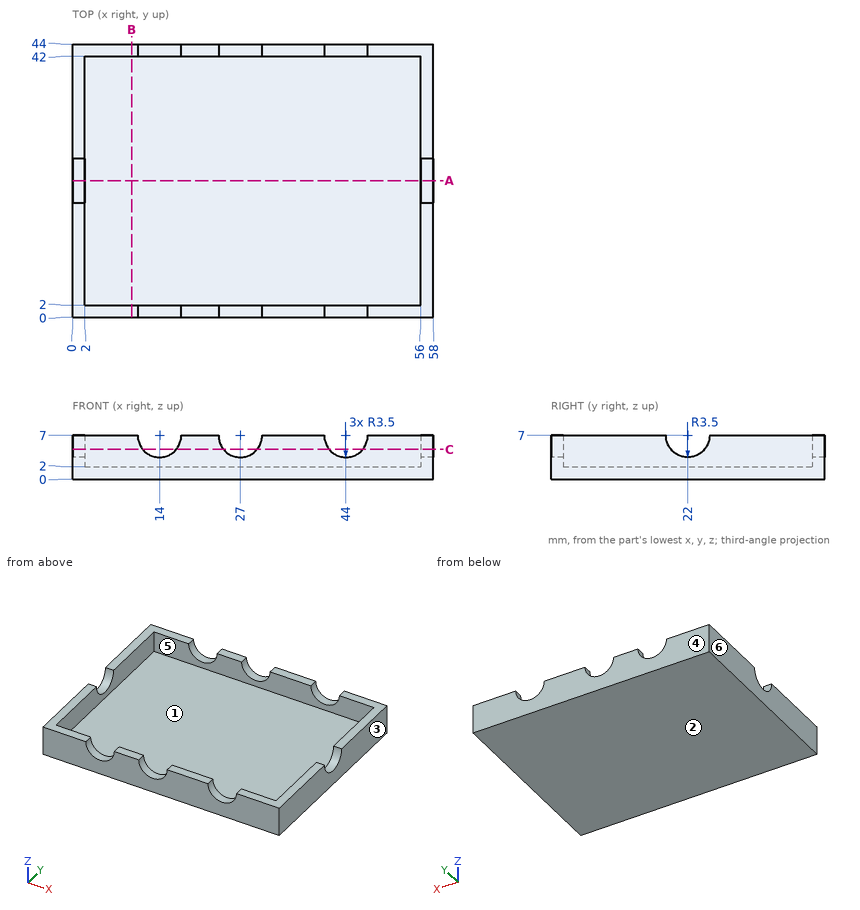
The drawing under review shows one solid part. Ordinate dimensions are in mm from its lowest x, y, z. A direction names the side the tool comes from. Coordinates: 2 decimals unless noted, no trailing zeros. Write each loop counter-clockwise with the first axis right and the second up, starting at its lowest first coordinate (ties: lowest second). Pieces come first, ordered by that corner, then holes. Notation, with made-up numbers: (-38.75, -16) - (7.25, -16) arc R21 ccw to (7.25, -6) - close; hole circle Ø10 at (52, -9). An arc over 180 degrees is marked (long way). Answer in a Markdown table with one row per item. Add a question column.
Q1. Draft analysis for pull direction X (two halves, no side actions). For the marked faces 3, 4, 5 and 6, state which applies: +X half, -X half, draft (parallel to the pull), parting line (faces both ways), or undercut.
Q2. We need section C-C, the plane z = 4.75. Count the separate pieces of the cut face and the enclosed holes in it, and give its area (3 significant figures).
Q3. We need section A-A, the plane y = 22. State the section outline as (x, z) points, and give its area (3 significant figures).
Q4. For P1, Ø1.5, axis at y = 22, z = 6, coming from the +X side; P2, Ø1, axis at x = 20.5, y = 27.5, coming from the +Z side, all flat-tipped, find the tip position at first contact; note any pin that passes through.
Q5. Tool access review of the marked faces 1 and 2: name each direction out of +Z, -Z, +X, -X, +Y, -Y from which nothing blocks a thin tool from reaching the whole face with its end or side.
Q6. For probe 1 along X at (y, z) = (28, 4); probe 2 along Y at (x, z) = (47.5, 6.25); probe 3 along Z at (x, y) = (45, 24), list the stretches that pass through material, from the lowest coordinate up.
Q7. We need section B-B, the plane x = 9.5. State the section outline as (y, z) points.
Answer list:
| question | item | result |
|---|---|---|
| 1 | face 3 | +X half |
| 1 | face 4 | draft |
| 1 | face 5 | undercut |
| 1 | face 6 | -X half |
| 2 | separate pieces | 8 |
| 2 | enclosed holes | 0 |
| 2 | area | 306 mm2 |
| 3 | outline | (0, 0) - (58, 0) - (58, 3.5) - (56, 3.5) - (56, 2) - (2, 2) - (2, 3.5) - (0, 3.5) - close |
| 3 | area | 122 mm2 |
| 4 | P1 | passes through |
| 4 | P2 | stops at z = 2 |
| 5 | face 1 | +Z |
| 5 | face 2 | -Z, +X, -X, +Y, -Y |
| 6 | probe 1 | x = 0 to 2, 56 to 58 |
| 6 | probe 2 | y = 0 to 2, 42 to 44 |
| 6 | probe 3 | z = 0 to 2 |
| 7 | outline | (0, 0) - (44, 0) - (44, 7) - (42, 7) - (42, 2) - (2, 2) - (2, 7) - (0, 7) - close |
